Check sheet for the modelled part. Datum: model origin and axes. Units: mm. A direction names the side the tool comes from. Give positions to 0.01 mm unless a question says otherwise; leave off trailing zeros. Loops run counter-clockwise (first coordinate to the right, second up) from the corner with the lowest first, then second, coordinate; pieces in that order, holes last. Notation, with made-up numbers: M 29,68 L 61,68 A25 cw 61,100 Z; hole C 82.5,80.5 d5. An arc over 180 degrees is marked long. Put each result on its own line as item: value. Start each with the question number.
```python
from build123d import *

# Parameters (mm, degrees)
F0_R           = 22.5
F1_DEPTH       = 10
F2_R           = 10
F3_DEPTH       = 10
F5_D           = 4.2
F5_CSINK_D     = 11.2
F5_CSINK_ANGLE = 90


with BuildPart() as f1:
    # F0 (on Front) → F1 (new body)
    with BuildSketch(Plane.XZ):
        Circle(F0_R)
    extrude(amount=F1_DEPTH)

    # F2 (on face) → F3 (join)
    with BuildSketch(Plane(origin=(0, 0, 0), x_dir=(-1, 0, 0), z_dir=(0, 1, 0))):
        Circle(F2_R)
    extrude(amount=F3_DEPTH)

    # F5 (through all)
    with Locations(Plane(origin=(0, 10, 0), x_dir=(-1, 0, 0), z_dir=(0, 1, 0))):
        with Locations((0, 0)):
            CounterSinkHole(F5_D / 2, F5_CSINK_D / 2, counter_sink_angle=F5_CSINK_ANGLE)


solid = f1.part
```
Q1. Thickness scan on line 1 along Z through (x, y) = (0, 1); line 2 along Z through (x, y) = (0, -1.25); line 3 along Y through (x, z) = (5, 12.5). Record the ranges inside material, lowest first. Write a range as [from, to].
Q2. Section check B-B, the plane x = 0. Record the cut outline in (y, z), then the cut area to 3 significant figures.
Q3. Section check C-C, the plane y = 5.25. Record the cut outline in (x, z).
Q4. Section check A-A, the plane z = 0. Record the cut outline in (x, y), then the cut area to 3 significant figures.
Q5. Depth check by flat-ended pin: P1, Ø1, axis at y = 2.5, z = 12, coming from the -X side; P2, Ø8, axis at x = 9, y = 4.5, coming from the -Z side; P3, Ø1, axis at x = 0, z = 17, coming from the +Y side; P4, Ø4, axis at y = 6.5, z = 0.5, coming from the +X side. Enter the tip coordinate at first touch or a pass-through.
Q6. Section check D-D, the plane x = 18. Record the cut outline in (y, z).
Q7. Mould release check, pull along X, two halves, no side actions. Record for faces 3 (the face through (10.382, -4.93, -19.961)), 4 (the face through (-0.492, 6.67, -2.216)), 5 (the face through (0, -10, -5)), 6 (the face through (2.003, -1.866, 0.631)): pulls with the +X half, pulls with the -X half, needs draft (parallel to the pull), parting line crosses it, or undercut.
Q8. Access from +Z, -Z, +X, -X, +Y, -Y to the whole of each face (thin tool, end or side, straight path). Record for faces 1 (the face through (5, 0, -10)), 2 (the face through (-4.3, 10, -4.3)).
Found:
1. line 1: z = [-10, -2.1], [2.1, 10]
1. line 2: z = [-22.5, -2.1], [2.1, 22.5]
1. line 3: y = [-10, 0]
2. outline: M -10,-22.5 L 0,-22.5 L 0,-10 L 10,-10 L 10,-5.6 L 6.5,-2.1 L -10,-2.1 Z; M -10,2.1 L 6.5,2.1 L 10,5.6 L 10,10 L 0,10 L 0,22.5 L -10,22.5 Z
2. area: 554 mm^2
3. outline: C 0,0 d20; hole C 0,0 d4.2
4. outline: M -22.5,-10 L -2.1,-10 L -2.1,6.5 L -5.6,10 L -10,10 L -10,0 L -22.5,0 Z; M 2.1,-10 L 22.5,-10 L 22.5,0 L 10,0 L 10,10 L 5.6,10 L 2.1,6.5 Z
4. area: 554 mm^2
5. P1: passes through
5. P2: stops at z = -8.66
5. P3: stops at y = 0
5. P4: stops at x = 10
6. outline: M -10,-13.5 L 0,-13.5 L 0,13.5 L -10,13.5 Z
7. face 3: parting line crosses it
7. face 4: undercut
7. face 5: needs draft
7. face 6: undercut
8. face 1: +Y
8. face 2: +Z, -Z, +X, -X, +Y
